Verification items for this drawing (mm, ordinates from the low corner). Give positions to 0.01 mm unless a question says otherwise; leave off trailing zeros. Write each loop counter-clockwise with the first axis right and the second up, starting at its lowest first coordinate (ties: lowest second). Pieces come first, ordered by that corner, then holes. Notation, with made-up numbers: (15.5, 19) -> (35.5, 19) arc R21 cw to (35.5, 44) -> close; hole circle Ø2 at (-33, 65). An arc over 180 degrees is marked (long way). Use one line per item in the form item = value. Start each with the question number.
(1) Section check B-B, the plane z = 1.9. Record the cut outline in (x, y) (1 decimal).
(2) Depth check by flat-ended pin: pin 1 Ø1.6 at (x, z) = (81, 2) entering from -Y (3 decimals). Enter the tip coordinate at first touch or a pass-through.
(3) Scan lines: L1, parallel to X at y = 2.25, z = 1.15 (3 decimals); L2, parallel to Y at x = 51, z = 2.5 (1 decimal). Record each from-to range of solid material in increasing order.
(4) Section check C-C, the plane x = 49.5. Record the cut outline in (y, z) (1 decimal).
(5) Section check A-A, the plane y = 2. Record the cut outline in (x, z) (3 decimals), plus the area to 3 significant figures.
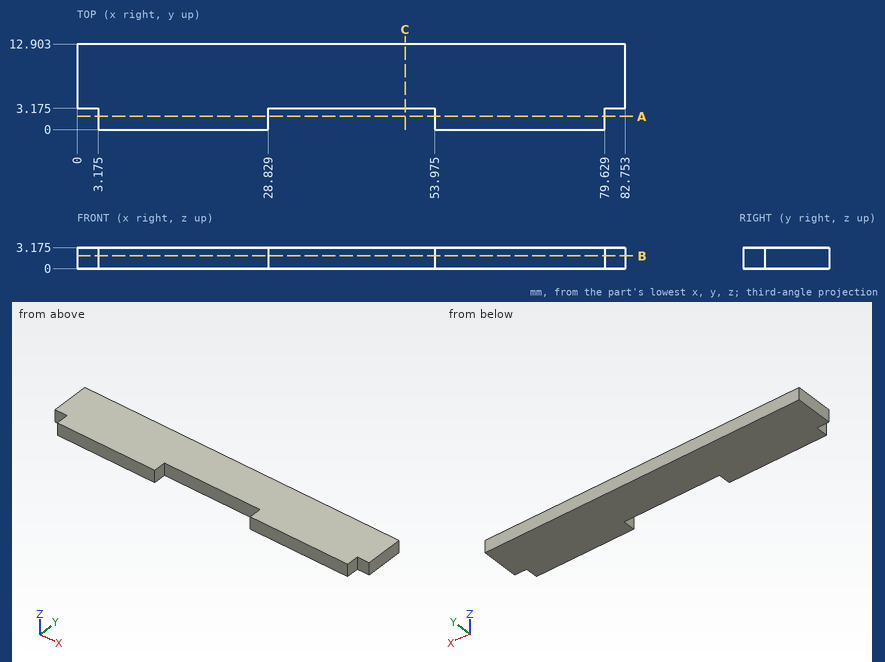
Completed:
q1.outline = (0, 3.2) -> (3.2, 3.2) -> (3.2, 0) -> (28.8, 0) -> (28.8, 3.2) -> (54, 3.2) -> (54, 0) -> (79.6, 0) -> (79.6, 3.2) -> (82.8, 3.2) -> (82.8, 12.9) -> (0, 12.9) -> close
q2.pin_1 = 3.175
q3.L1 = 3.175 to 28.829, 53.975 to 79.629
q3.L2 = 3.2 to 12.9
q4.outline = (3.2, 0) -> (12.9, 0) -> (12.9, 3.2) -> (3.2, 3.2) -> close
q5.outline = (3.175, 0) -> (28.829, 0) -> (28.829, 3.175) -> (3.175, 3.175) -> close; (53.975, 0) -> (79.629, 0) -> (79.629, 3.175) -> (53.975, 3.175) -> close
q5.area = 163 mm²
